from build123d import *
from build123d.topology import SkipClean

# Parameters (mm, degrees)
SKETCH_1_W                = 40
SKETCH_1_H                = 40
SKETCH_1_R                = 1.55
EXTRUDE_2_DEPTH           = 3
CUT_EXTRUDE_1_DEPTH       = 1.5
SKETCH_2_W                = 3
SKETCH_2_H                = 3
EXTRUDE_7_DEPTH           = 45
SKETCH_5_W                = 40
SKETCH_5_H                = 3
EXTRUDE_8_DEPTH           = 40
SKETCH_6_R                = 12.5
CUT_EXTRUDE_2_DEPTH       = 4
CUT_EXTRUDE_START         = -4
CUT_EXTRUDE_3_DEPTH       = 4
SKETCH_8_R                = 5
CUT_EXTRUDE_4_DEPTH       = 4
SKETCH_9_R                = 2.5
CUT_EXTRUDE_5_DEPTH       = 4
SKETCH_10_W               = 1.5
SKETCH_10_H               = 34
SKETCH_10_W_2             = 34
SKETCH_10_H_2             = 1.5
EXTRUDE_10_DEPTH          = 45
CUT_EXTRUDE_12_DEPTH      = 63.507999488
CUT_EXTRUDE_12_DEPTH_BACK = 4
CUT_EXTRUDE_13_DEPTH      = 4
CUT_EXTRUDE_13_DEPTH_BACK = 64.442887702
CUT_EXTRUDE_15_DEPTH      = 10
CUT_EXTRUDE_15_DEPTH_BACK = 64.442887702
SKETCH_24_5_R             = 1.85
SKETCH_24_5_R_2           = 5.5
CUT_EXTRUDE_16_DEPTH      = 10
CUT_EXTRUDE_16_DEPTH_BACK = 64.442887702
SKETCH_25_R               = 5.5
SKETCH_25_R_2             = 1.85
SKETCH_26_W               = 40
SKETCH_26_H               = 40
CUT_EXTRUDE_17_DEPTH      = 54.150729064
EXTRUDE_START             = -3
SKETCH_27_R               = 5
SKETCH_27_R_2             = 2.1
EXTRUDE_12_DEPTH          = 3


with BuildPart() as part:
    # Sketch 1 → Extrude 2 (new body)
    with BuildSketch(Plane(origin=(0, 0, 0), x_dir=(1, 0, 0), z_dir=(0, 1, 0))):
        Rectangle(SKETCH_1_W, SKETCH_1_H)
        with Locations(Location((0, 8.5, 0), (0, 0, 270))):
            Circle(SKETCH_1_R, mode=Mode.SUBTRACT)
        with Locations(Location((8.5, 0, 0), (0, 0, 270))):
            Circle(SKETCH_1_R, mode=Mode.SUBTRACT)
        with Locations(Location((0, -8.5, 0), (0, 0, 270))):
            Circle(SKETCH_1_R, mode=Mode.SUBTRACT)
        with Locations(Location((-8.5, 0, 0), (0, 0, 270))):
            Circle(SKETCH_1_R, mode=Mode.SUBTRACT)
    extrude(amount=-EXTRUDE_2_DEPTH)

    # Sketch 1_6 → Cut-Extrude 1 (cut)
    with BuildSketch(Plane(origin=(0, 0, 0), x_dir=(1, 0, 0), z_dir=(0, 1, 0))):
        with BuildLine():
            ThreePointArc((4, 0), (2.828427125, 2.828427125), (0, 4))
            Line((0, 4), (0, -4))
            ThreePointArc((0, -4), (2.828427125, -2.828427125), (4, 0))
        make_face()
        with BuildLine():
            Line((0, -4), (0, 4))
            ThreePointArc((0, 4), (-4, 0), (0, -4))
        make_face()
    extrude(amount=-CUT_EXTRUDE_1_DEPTH, mode=Mode.SUBTRACT)

    # Sketch 2 → Extrude 7 (add)
    with BuildSketch(Plane(origin=(0, 0, 0), x_dir=(1, 0, 0), z_dir=(0, 1, 0))):
        with Locations((-18.5, 18.5)):
            Rectangle(SKETCH_2_W, SKETCH_2_H)
        with Locations((18.5, 18.5)):
            Rectangle(SKETCH_2_W, SKETCH_2_H)
        with Locations((18.5, -18.5)):
            Rectangle(SKETCH_2_W, SKETCH_2_H)
        with Locations((-18.5, -18.5)):
            Rectangle(SKETCH_2_W, SKETCH_2_H)
    extrude(amount=EXTRUDE_7_DEPTH)

    # Sketch 5 → Extrude 8 (add)
    with BuildSketch(Plane.ZY.offset(20)):
        with Locations((0, 43.5)):
            Rectangle(SKETCH_5_W, SKETCH_5_H)
    extrude(amount=-EXTRUDE_8_DEPTH)

    # Sketch 6 → Cut-Extrude 2 (cut)
    with BuildSketch(Plane(origin=(0, 45, 0), x_dir=(1, 0, 0), z_dir=(0, 1, 0))):
        with Locations(Location((0, 0, 0), (0, 0, 270))):
            Circle(SKETCH_6_R)
    extrude(amount=-CUT_EXTRUDE_2_DEPTH, mode=Mode.SUBTRACT)

    # Sketch 7 → Cut-Extrude 3 (cut)
    with SkipClean():  # the faces are left unmerged after this step: merging them gives an invalid solid
        with BuildSketch(Plane.XZ.offset(3).offset(CUT_EXTRUDE_START)):
            with BuildLine():
                ThreePointArc((-4, 0), (-2.828427125, -2.828427125), (0, -4))
                Line((0, -4), (0, 0))
                Line((0, 0), (-4, 0))
            make_face()
            with BuildLine():
                Line((0, 0), (0, -4))
                ThreePointArc((0, -4), (2.828427125, -2.828427125), (4, 0))
                ThreePointArc((4, 0), (0, 4), (-4, 0))
                Line((-4, 0), (0, 0))
            make_face()
        extrude(amount=CUT_EXTRUDE_3_DEPTH, mode=Mode.SUBTRACT)

    # Sketch 8 → Cut-Extrude 4 (cut)
    with SkipClean():  # the faces are left unmerged after this step: merging them gives an invalid solid
        with BuildSketch(Plane.XZ.offset(3)):
            with Locations(Location((-12, 12, 0), (0, 0, 270))):
                Circle(SKETCH_8_R)
            with Locations(Location((12, 12, 0), (0, 0, 270))):
                Circle(SKETCH_8_R)
            with Locations(Location((12, -12, 0), (0, 0, 270))):
                Circle(SKETCH_8_R)
            with Locations(Location((-12, -12, 0), (0, 0, 270))):
                Circle(SKETCH_8_R)
        extrude(amount=-CUT_EXTRUDE_4_DEPTH, mode=Mode.SUBTRACT)

    # Sketch 9 → Cut-Extrude 5 (cut)
    with SkipClean():  # the faces are left unmerged after this step: merging them gives an invalid solid
        with BuildSketch(Plane(origin=(0, 45, 0), x_dir=(1, 0, 0), z_dir=(0, 1, 0))):
            with Locations(Location((-12.727922061, 12.727922061, 0), (0, 0, 270))):
                Circle(SKETCH_9_R)
            with Locations(Location((12.727922061, 12.727922061, 0), (0, 0, 270))):
                Circle(SKETCH_9_R)
            with Locations(Location((12.727922061, -12.727922061, 0), (0, 0, 270))):
                Circle(SKETCH_9_R)
            with Locations(Location((-12.727922061, -12.727922061, 0), (0, 0, 270))):
                Circle(SKETCH_9_R)
        extrude(amount=-CUT_EXTRUDE_5_DEPTH, mode=Mode.SUBTRACT)

    # Sketch 10 → Extrude 10 (add)
    with SkipClean():  # the faces are left unmerged after this step: merging them gives an invalid solid
        with BuildSketch(Plane(origin=(0, 0, 0), x_dir=(1, 0, 0), z_dir=(0, 1, 0))):
            with Locations((19.25, 0)):
                Rectangle(SKETCH_10_W, SKETCH_10_H)
            with Locations((0, -19.25)):
                Rectangle(SKETCH_10_W_2, SKETCH_10_H_2)
            with Locations((-19.25, 0)):
                Rectangle(SKETCH_10_W, SKETCH_10_H)
            with Locations((0, 19.25)):
                Rectangle(SKETCH_10_W_2, SKETCH_10_H_2)
        extrude(amount=EXTRUDE_10_DEPTH)

    # Sketch 20 → Cut-Extrude 12 (cut, two sides: drawn at the far end of the back side and taken through both)
    with SkipClean():  # the faces are left unmerged after this step: merging them gives an invalid solid
        with BuildSketch(Plane(origin=(0, 0, 18.5), x_dir=(-1, 0, 0), z_dir=(0, 0, -1)).offset(-CUT_EXTRUDE_12_DEPTH_BACK)):
            with BuildLine():
                Line((-2.45, 36.5), (-2.45, 5.5))
                ThreePointArc((-2.45, 5.5), (0, 3.05), (2.45, 5.5))
                Line((2.45, 5.5), (2.45, 36.5))
                ThreePointArc((2.45, 36.5), (0, 38.95), (-2.45, 36.5))
            make_face()
        extrude(amount=CUT_EXTRUDE_12_DEPTH + CUT_EXTRUDE_12_DEPTH_BACK, mode=Mode.SUBTRACT)

    # Sketch 24 → Cut-Extrude 13 (cut, two sides: drawn at the far end of the back side and taken through both)
    with SkipClean():  # the faces are left unmerged after this step: merging them gives an invalid solid
        with BuildSketch(Plane(origin=(20, 0, 0), x_dir=(0, 0, -1), z_dir=(1, 0, 0)).offset(-CUT_EXTRUDE_13_DEPTH_BACK)):
            with BuildLine():
                Line((-2.45, 36.5), (-2.45, 5.5))
                ThreePointArc((-2.45, 5.5), (0, 3.05), (2.45, 5.5))
                Line((2.45, 5.5), (2.45, 36.5))
                ThreePointArc((2.45, 36.5), (0, 38.95), (-2.45, 36.5))
            make_face()
        extrude(amount=CUT_EXTRUDE_13_DEPTH + CUT_EXTRUDE_13_DEPTH_BACK, mode=Mode.SUBTRACT)

    # Sketch 24_5 → Cut-Extrude 15 (cut, two sides: drawn at the far end of the back side and taken through both)
    with SkipClean():  # the faces are left unmerged after this step: merging them gives an invalid solid
        with BuildSketch(Plane(origin=(20, 0, 0), x_dir=(0, 0, -1), z_dir=(1, 0, 0)).offset(-CUT_EXTRUDE_15_DEPTH_BACK)):
            with Locations((-11.45, 35)):
                Circle(SKETCH_24_5_R)
            with Locations(Location((-11.45, 7, 0), (0, 0, 180))):
                Circle(SKETCH_24_5_R)
            with Locations((11.45, 7)):
                Circle(SKETCH_24_5_R)
            with Locations(Location((11.45, 35, 0), (0, 0, 180))):
                Circle(SKETCH_24_5_R)
            with Locations((-11.35, 21)):
                Circle(SKETCH_24_5_R_2)
            with Locations(Location((11.35, 21, 0), (0, 0, 180))):
                Circle(SKETCH_24_5_R_2)
        extrude(amount=CUT_EXTRUDE_15_DEPTH + CUT_EXTRUDE_15_DEPTH_BACK, mode=Mode.SUBTRACT)

    # Sketch 25 → Cut-Extrude 16 (cut, two sides: drawn at the far end of the back side and taken through both)
    with SkipClean():  # the faces are left unmerged after this step: merging them gives an invalid solid
        with BuildSketch(Plane(origin=(0, 0, -20), x_dir=(-1, 0, 0), z_dir=(0, 0, -1)).offset(-CUT_EXTRUDE_16_DEPTH_BACK)):
            with Locations((-11.45, 21)):
                Circle(SKETCH_25_R)
            with Locations((11.45, 21)):
                Circle(SKETCH_25_R)
            with Locations((-11.45, 35)):
                Circle(SKETCH_25_R_2)
            with Locations((-11.45, 7)):
                Circle(SKETCH_25_R_2)
            with Locations((11.45, 7)):
                Circle(SKETCH_25_R_2)
            with Locations((11.45, 35)):
                Circle(SKETCH_25_R_2)
        extrude(amount=CUT_EXTRUDE_16_DEPTH + CUT_EXTRUDE_16_DEPTH_BACK, mode=Mode.SUBTRACT)

    # Sketch 26 → Cut-Extrude 17 (cut, through all)
    with SkipClean():  # the faces are left unmerged after this step: merging them gives an invalid solid
        with BuildSketch(Plane(origin=(0, 0, 0), x_dir=(1, 0, 0), z_dir=(0, 1, 0))):
            Rectangle(SKETCH_26_W, SKETCH_26_H)
        extrude(amount=CUT_EXTRUDE_17_DEPTH, mode=Mode.SUBTRACT)

    # Sketch 27 → Extrude 12 (add)
    # profile 1 of 4: a face of its own
    with SkipClean():  # the faces are left unmerged after this step: merging them gives an invalid solid
        with BuildSketch(Plane(origin=(0, 0, 0), x_dir=(1, 0, 0), z_dir=(0, 1, 0)).offset(EXTRUDE_START)):
            with Locations((-12, 12)):
                Circle(SKETCH_27_R)
            with Locations(Location((-12, 12, 0), (0, 0, 270))):
                Circle(SKETCH_27_R_2, mode=Mode.SUBTRACT)
        # profile 2 of 4: a face of its own
        with BuildSketch(Plane(origin=(0, 0, 0), x_dir=(1, 0, 0), z_dir=(0, 1, 0)).offset(EXTRUDE_START)):
            with Locations((12, 12)):
                Circle(SKETCH_27_R)
            with Locations(Location((12, 12, 0), (0, 0, 270))):
                Circle(SKETCH_27_R_2, mode=Mode.SUBTRACT)
        # profile 3 of 4: a face of its own
        with BuildSketch(Plane(origin=(0, 0, 0), x_dir=(1, 0, 0), z_dir=(0, 1, 0)).offset(EXTRUDE_START)):
            with Locations((-12, -12)):
                Circle(SKETCH_27_R)
            with Locations(Location((-12, -12, 0), (0, 0, 270))):
                Circle(SKETCH_27_R_2, mode=Mode.SUBTRACT)
        # profile 4 of 4: a face of its own
        with BuildSketch(Plane(origin=(0, 0, 0), x_dir=(1, 0, 0), z_dir=(0, 1, 0)).offset(EXTRUDE_START)):
            with Locations((12, -12)):
                Circle(SKETCH_27_R)
            with Locations(Location((12, -12, 0), (0, 0, 270))):
                Circle(SKETCH_27_R_2, mode=Mode.SUBTRACT)
        extrude(amount=EXTRUDE_12_DEPTH)


solid = part.part
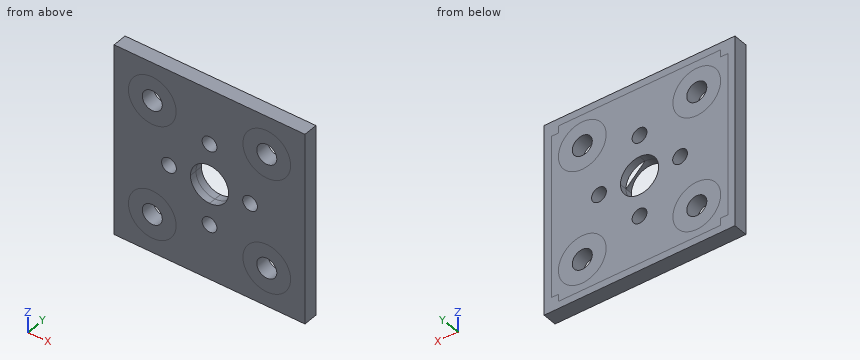
Model file for the job. Use its own axes, mm. Round coordinates to 2 decimals unless told otherwise and drop trailing zeros. Order: outer loops, then holes, each group sorted by start corner. A loop starts at its lowest first (then second) coordinate and runs counter-clockwise, first axis right, second up. Notation, with made-up numbers: M 74,-15.5 L 132,-15.5 A34 ccw 132,17.5 Z; hole C 73,51 d10. An arc over 180 degrees is marked long. Write each question's results on one line, items separated by ' | '. Start each with the question number.
(1) Drop a flat-ended pin along its axis: pin 1 (6.5 mm diameter, centred on x = -12, z = 12, fed in from +Y). Give the stop position or say it passes through.
(2) Probe probe 1 along X at (y, z) = (-1.9, 0); probe 2 along X at (y, z) = (-1.45, -11.5). List the from-to ranges inside material, lowest first. Write a range as from..to.
(3) Saw through at A-A, the plane z = -8.5. Give the cut face in (x, y), then the cut area to 3 significant figures.
(4) Saw through at C-C, the plane y = -0.85. State how many separate pieces and enclosed holes the cut face has, then the cut area to 3 significant figures.
(5) Saw through at D-D, the plane z = 11.5. Give the cut face in (x, y).
(6) Saw through at B-B, the plane x = 12. Give the cut face in (y, z), then the cut area to 3 significant figures.
Established:
1) pin 1: stops at y = 0
2) probe 1: x = -20..-10.05, -6.95..-4, 4..6.95, 10.05..20 | probe 2: x = -20..-14.04, -9.96..9.96, 14.04..20
3) outline: M -20,-3 L -1.55,-3 L -1.55,0 L -20,0 Z; M 1.55,-3 L 20,-3 L 20,0 L 1.55,0 Z | area: 111 mm^2
4) separate pieces: 1 | enclosed holes: 9 | area: 1,460 mm^2
5) outline: M -20,-3 L -14.04,-3 L -14.04,0 L -20,0 Z; M -9.96,-3 L 9.96,-3 L 9.96,0 L -9.96,0 Z; M 14.04,-3 L 20,-3 L 20,0 L 14.04,0 Z
6) outline: M -3,-20 L 0,-20 L 0,-14.1 L -3,-14.1 Z; M -3,-9.9 L 0,-9.9 L 0,9.9 L -3,9.9 Z; M -3,14.1 L 0,14.1 L 0,20 L -3,20 Z | area: 94.8 mm^2
